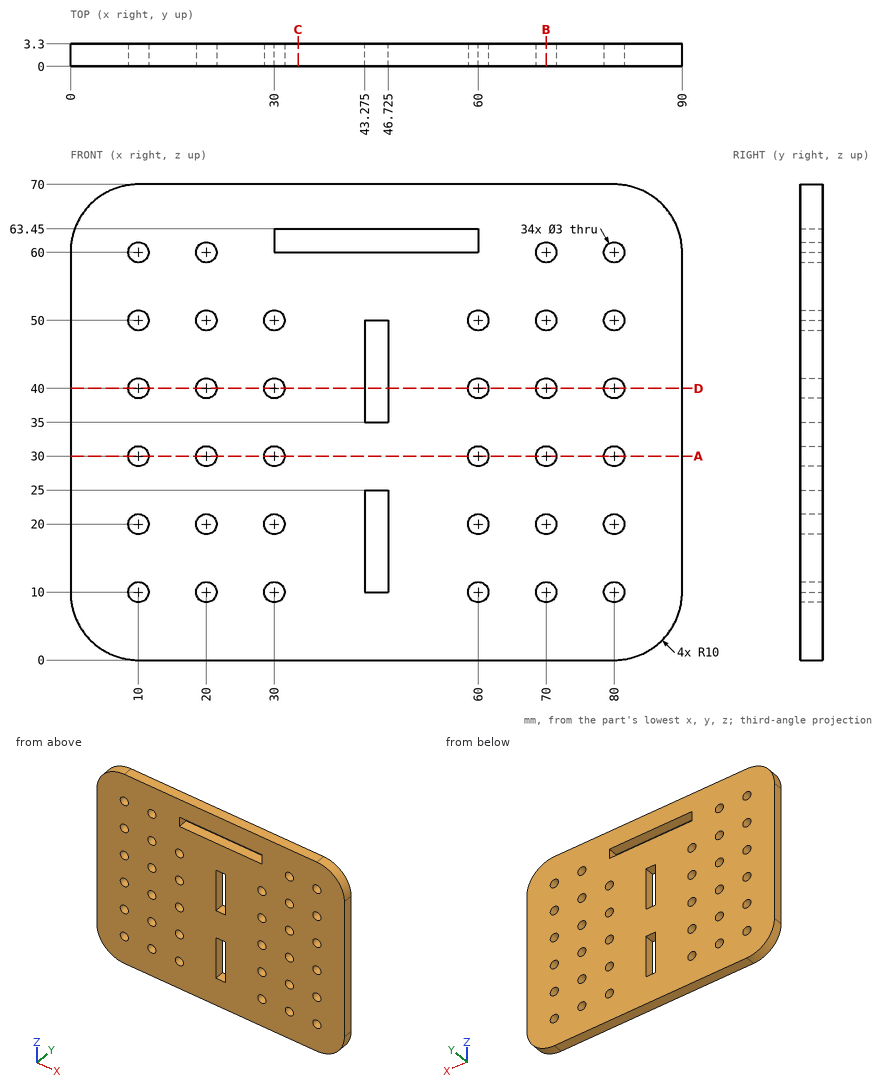
Check sheet for the drawn part. Datum: minimum x, y, z corner. Units: mm. Coordinates: 2 decimals unless noted, no trailing zeros. Write each loop counter-clockwise with the first axis right and the second up, starting at its lowest first coordinate (ties: lowest second). Pieces come first, ordered by that corner, then holes. Notation, with made-up numbers: (60.25, 47) - (79.25, 47) arc R29 cw to (79.25, 72) - close; hole circle Ø1 at (-14, 63). An arc over 180 degrees is marked (long way). Answer as a JSON object with one key per item and string values.
(1) Cross-section at B-B on x = 70. Record the cut outline in (y, z).
Report:
{"outline": "(0, 0) - (3.3, 0) - (3.3, 8.5) - (0, 8.5) - close; (0, 11.5) - (3.3, 11.5) - (3.3, 18.5) - (0, 18.5) - close; (0, 21.5) - (3.3, 21.5) - (3.3, 28.5) - (0, 28.5) - close; (0, 31.5) - (3.3, 31.5) - (3.3, 38.5) - (0, 38.5) - close; (0, 41.5) - (3.3, 41.5) - (3.3, 48.5) - (0, 48.5) - close; (0, 51.5) - (3.3, 51.5) - (3.3, 58.5) - (0, 58.5) - close; (0, 61.5) - (3.3, 61.5) - (3.3, 70) - (0, 70) - close"}
(2) Thickness scan on line 1 along Z through (x, y) = (44, 1.9); line 2 along X through (y, z) = (1.25, 47.5) (3 decimals); line 3 along X through (y, z) = (2.15, 63). Record the ranges inside material, lowest first.
Report:
{"line 1": "0 to 10, 25 to 35, 50 to 60, 63.45 to 70", "line 2": "0 to 43.275, 46.725 to 90", "line 3": "0.46 to 30, 60 to 89.54"}
(3) Cross-section at C-C on x = 33.5. Record the cut outline in (y, z).
Report:
{"outline": "(0, 0) - (3.3, 0) - (3.3, 60) - (0, 60) - close; (0, 63.45) - (3.3, 63.45) - (3.3, 70) - (0, 70) - close"}
(4) Cross-section at A-A on z = 30. Record the cut outline in (x, y), plus the area to 3 significant figures.
Report:
{"outline": "(0, 0) - (8.5, 0) - (8.5, 3.3) - (0, 3.3) - close; (11.5, 0) - (18.5, 0) - (18.5, 3.3) - (11.5, 3.3) - close; (21.5, 0) - (28.5, 0) - (28.5, 3.3) - (21.5, 3.3) - close; (31.5, 0) - (58.5, 0) - (58.5, 3.3) - (31.5, 3.3) - close; (61.5, 0) - (68.5, 0) - (68.5, 3.3) - (61.5, 3.3) - close; (71.5, 0) - (78.5, 0) - (78.5, 3.3) - (71.5, 3.3) - close; (81.5, 0) - (90, 0) - (90, 3.3) - (81.5, 3.3) - close", "area": "238 mm^2"}
(5) Cross-section at D-D on z = 40. Give the number of separate pieces and of enclosed holes in the cut face, plus the area to 3 significant figures.
Report:
{"separate pieces": "8", "enclosed holes": "0", "area": "226 mm^2"}
